from build123d import *

# Parameters (mm, degrees)
RESSALTO_EXTRUS_O1_DEPTH = 2
ESBO_O4_R                = 2.5
RESSALTO_EXTRUS_O2_DEPTH = 2
ESBO_O2_R                = 0.85
CORTE_EXTRUS_O1_DEPTH    = 17.680827318
CORTE_EXTRUS_O2_REACH    = 18.317
ESBO_O3_R                = 0.5
RESSALTO_EXTRUS_O3_DEPTH = 0.5


with BuildPart() as part:
    # Esboço1 → Ressalto-extrusão1 (new body)
    with BuildSketch(Plane(origin=(0, 0, 0), x_dir=(1, 0, 0), z_dir=(0, 1, 0))):
        with BuildLine():
            Line((-13.5, 2.5), (13.5, 2.5))
            ThreePointArc((13.5, 2.5), (16, 0), (13.5, -2.5))
            Line((13.5, -2.5), (-13.5, -2.5))
            ThreePointArc((-13.5, -2.5), (-16, 0), (-13.5, 2.5))
        make_face()
    extrude(amount=RESSALTO_EXTRUS_O1_DEPTH)

    # Esboço4 → Ressalto-extrusão2 (add)
    with BuildSketch(Plane(origin=(0, 2, 0), x_dir=(1, 0, 0), z_dir=(0, 1, 0))):
        with Locations(Location((-13.5, 0, 0), (0, 0, 270))):
            Circle(ESBO_O4_R)
    extrude(amount=RESSALTO_EXTRUS_O2_DEPTH)

    # Esboço2 → Corte-extrusão1 (cut, through all)
    with BuildSketch(Plane(origin=(0, 4, 0), x_dir=(1, 0, 0), z_dir=(0, 1, 0))):
        with Locations(Location((-13.5, 0, 0), (0, 0, 270))):
            Circle(ESBO_O2_R)
    extrude(amount=-CORTE_EXTRUS_O1_DEPTH, mode=Mode.SUBTRACT)

    # Esboço3 → Corte-extrusão2 (cut, up to next)
    with BuildSketch(Plane(origin=(0, 2, 0), x_dir=(1, 0, 0), z_dir=(0, 1, 0)), mode=Mode.PRIVATE) as corte_extrus_o2_sk1:
        with Locations(Location((13.5, 0, 0), (0, 0, 270))):
            Circle(ESBO_O3_R)
    corte_extrus_o2_tool1 = extrude(corte_extrus_o2_sk1.sketch, amount=-CORTE_EXTRUS_O2_REACH, mode=Mode.PRIVATE) & part.part
    add(corte_extrus_o2_tool1.solids().sort_by_distance((13.5, 2, 0))[0], mode=Mode.SUBTRACT)

    # Esboço5 → Ressalto-extrusão3 (add)
    with BuildSketch(Plane(origin=(0, 2, 0), x_dir=(1, 0, 0), z_dir=(0, 1, 0))):
        with BuildLine():
            Line((-10.245767212, -1), (-10.245767212, 1))
            Line((-10.245767212, 1), (-9.841921058, 1))
            add(Edge.make_bspline(
                [(-9.841921058, 1), (-9.806795922, 0.999747103), (-9.738934342, 0.999258507), (-9.640870086, 0.996160569), (-9.550136507, 0.990680303), (-9.467032017, 0.982697717), (-9.391328467, 0.972895983), (-9.323237834, 0.960610038), (-9.262408038, 0.946102512), (-9.224996929, 0.933733683), (-9.207305673, 0.927884615)],
                knots=[0, 0, 0, 0, 1.314313732, 2.53924729, 3.670748893, 4.714932338, 5.66265055, 6.526160246, 7.303039223, 8, 8, 8, 8], degree=3))
            add(Edge.make_bspline(
                [(-9.207305673, 0.927884615), (-9.184165822, 0.919067069), (-9.138410855, 0.90163193), (-9.073263928, 0.868742615), (-9.011935149, 0.831477985), (-8.954095638, 0.789788921), (-8.901066594, 0.742495007), (-8.850776368, 0.691605244), (-8.80528224, 0.63526905), (-8.763620356, 0.574654771), (-8.726057122, 0.510476455), (-8.693406175, 0.442856393), (-8.666289607, 0.372137989), (-8.643779192, 0.298517904), (-8.626038359, 0.22183426), (-8.613934398, 0.141997765), (-8.605950975, 0.059323942), (-8.60514866, 0.003224249), (-8.604741571, -0.025240385)],
                knots=[0, 0, 0, 0, 0.984719456, 1.947108742, 2.898477687, 3.838006223, 4.779231079, 5.722358779, 6.681677486, 7.655904652, 8.64651281, 9.637519902, 10.640069247, 11.656948941, 12.698408672, 13.768548281, 14.867775369, 16, 16, 16, 16], degree=3))
            add(Edge.make_bspline(
                [(-8.604741571, -0.025240385), (-8.605100981, -0.049961092), (-8.605809236, -0.098675829), (-8.612168845, -0.170470626), (-8.621412456, -0.240135524), (-8.635723426, -0.307338781), (-8.653096291, -0.372669192), (-8.675361521, -0.435430474), (-8.700867518, -0.496198365), (-8.730610306, -0.554151209), (-8.763262526, -0.609055993), (-8.798303522, -0.660813437), (-8.83569592, -0.708684993), (-8.875796281, -0.752815628), (-8.918086405, -0.793138816), (-8.962843165, -0.829991396), (-9.010182051, -0.862652284), (-9.059891036, -0.892404918), (-9.113420253, -0.918359407), (-9.171783605, -0.940319412), (-9.235229992, -0.958517478), (-9.303603682, -0.973700847), (-9.377022812, -0.98574502), (-9.455559364, -0.993817244), (-9.539092672, -0.999276063), (-9.596452252, -0.999754002), (-9.625975545, -1)],
                knots=[0, 0, 0, 0, 1.105936401, 2.179363191, 3.223086493, 4.248585256, 5.251745608, 6.245858792, 7.225916811, 8.198733463, 9.158002045, 10.082870192, 10.993790845, 11.873723703, 12.748670949, 13.606408763, 14.465103618, 15.319838547, 16.196477973, 17.123216899, 18.106603292, 19.147568657, 20.255746949, 21.433717677, 22.679120308, 24, 24, 24, 24], degree=3))
            Line((-9.625975545, -1), (-10.245767212, -1))
        make_face()
        with BuildLine():
            Line((-10.066280032, -0.794871795), (-9.836712725, -0.794871795))
            add(Edge.make_bspline(
                [(-9.836712725, -0.794871795), (-9.803725084, -0.794730026), (-9.740277771, -0.794457351), (-9.64904463, -0.792064664), (-9.565684974, -0.788154985), (-9.490186969, -0.782683512), (-9.422593241, -0.775444303), (-9.362762527, -0.76737293), (-9.31089095, -0.757317244), (-9.279502701, -0.74820241), (-9.264997981, -0.743990385)],
                knots=[0, 0, 0, 0, 1.375205317, 2.645023457, 3.804390687, 4.853969522, 5.800190428, 6.637939096, 7.370582563, 8, 8, 8, 8], degree=3))
            add(Edge.make_bspline(
                [(-9.264997981, -0.743990385), (-9.246741774, -0.737560923), (-9.21066541, -0.724855567), (-9.158733361, -0.70167976), (-9.110300787, -0.674227149), (-9.064523629, -0.643711564), (-9.022051255, -0.609056706), (-8.982380331, -0.57101614), (-8.945590731, -0.529396269), (-8.912062555, -0.484248748), (-8.882057809, -0.435854579), (-8.85607425, -0.384689531), (-8.833301946, -0.331314211), (-8.815428464, -0.274908978), (-8.801419559, -0.215978087), (-8.79149688, -0.154517394), (-8.785317038, -0.090538376), (-8.78459621, -0.047022876), (-8.78422875, -0.024839744)],
                knots=[0, 0, 0, 0, 0.998632004, 1.973411704, 2.929992603, 3.868527914, 4.809262121, 5.754881198, 6.702106254, 7.672490631, 8.653608572, 9.636854334, 10.631411391, 11.644891563, 12.686317036, 13.754757253, 14.855430412, 16, 16, 16, 16], degree=3))
            add(Edge.make_bspline(
                [(-8.78422875, -0.024839744), (-8.784522057, -0.001449183), (-8.785098262, 0.044501779), (-8.792340725, 0.111925034), (-8.802924471, 0.17677112), (-8.818229434, 0.239044374), (-8.837732794, 0.29886629), (-8.862072589, 0.35590601), (-8.889882086, 0.410765935), (-8.922969707, 0.462179858), (-8.959207189, 0.510804492), (-8.99942312, 0.555350158), (-9.04297857, 0.595918329), (-9.089398484, 0.633140794), (-9.139991112, 0.665520037), (-9.19356465, 0.694483855), (-9.250905033, 0.719064364), (-9.290798003, 0.732138), (-9.311071699, 0.738782051)],
                knots=[0, 0, 0, 0, 1.122418816, 2.205001699, 3.251619955, 4.274784885, 5.280384055, 6.268708349, 7.249350384, 8.229342522, 9.199999885, 10.157847722, 11.105861043, 12.055065948, 13.010012805, 13.98527497, 14.976112212, 16, 16, 16, 16], degree=3))
            add(Edge.make_bspline(
                [(-9.311071699, 0.738782051), (-9.327843783, 0.74342001), (-9.363505834, 0.753281583), (-9.421699814, 0.764038939), (-9.487194185, 0.773527224), (-9.560279728, 0.781560389), (-9.640873134, 0.787324573), (-9.729036384, 0.791651038), (-9.824807586, 0.794569114), (-9.891197606, 0.794768375), (-9.925655032, 0.794871795)],
                knots=[0, 0, 0, 0, 0.674548936, 1.434276114, 2.292660221, 3.240891867, 4.284742987, 5.42552168, 6.663806718, 8, 8, 8, 8], degree=3))
            Line((-9.925655032, 0.794871795), (-10.066280032, 0.794871795))
            Line((-10.066280032, 0.794871795), (-10.066280032, -0.794871795))
        make_face(mode=Mode.SUBTRACT)
    extrude(amount=RESSALTO_EXTRUS_O3_DEPTH)


solid = part.part
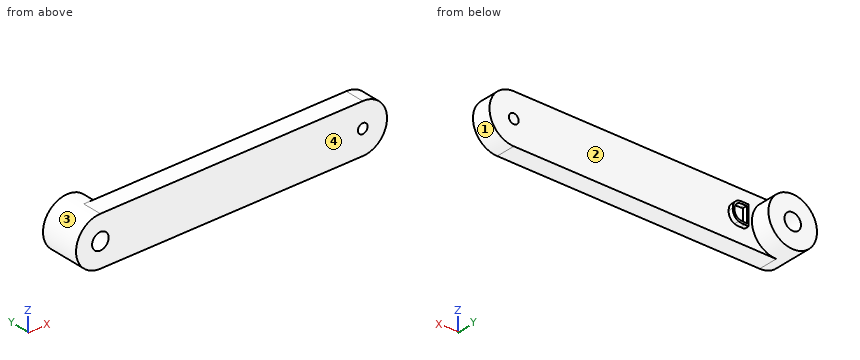
Input: part model. Units: mm. Frame: model coordinates. Face numbers are marked on the shaded views. A direction names the side the tool comes from. Give positions to 0.01 mm unless a question says otherwise; leave off trailing zeros. Loops run counter-clockwise (first coordinate to the right, second up) from the corner with the lowest first, then second, coordinate; pieces in that order, holes last. Notation, with made-up numbers: (-17, 56.5) -> (-4, 56.5) arc R30 cw to (-4, 89.5) -> close; hole circle Ø7 at (77, 46.25). An arc over 180 degrees is marked (long way). Answer as a JSON object with one key per item and string values. Group by question number.
Item 1: Cut plane A-A, the plane y = 1.3. Return the cut outline in (x, z), and give its area (3 significant figures).
Item 2: Reachability of the marked faces 3 and 4 from +Z, -Z, +X, -X, +Y, -Y: full face, straight path, thin tool, end or side. Return the list, or none.
Item 3: Pull-direction query (Z, two-part tool) for the marked faces 1 and 2; classes: released by +Z, released by -Z, zero draft, split by the parting line, or undercut.
Item 4: Line query: probe 1 along X at (y, z) = (2.25, 0); probe 2 along X at (y, z) = (1.7, 0); probe 3 along X at (y, z) = (3.25, 0). Output: solid intervals per line, ascending.
Item 5: Cut plane B-B, the plane z = 1.3. Return the cut outline in (x, y), and give its area (3 significant figures).
Item 6: Cut plane C-C, the plane y = 3.35. Return the cut outline in (x, z).
Item 7: Cut plane D-D, the plane x = -6. Return the cut outline in (y, z), and give its area (3 significant figures).
Item 8: Pin query (flat end, axial travel): P1, Ø1, axis at x = -9.5, z = 0, coming from the +Y side; P2, Ø1.8, axis at x = -9.5, z = 0.5, coming from the +Y side. Return the tip coordinate at first contact, or that it passes through.
Checks:
{
 "1": {"outline": "(-13.5, -2.5) -> (13.5, -2.5) arc R2.5 ccw to (13.5, 2.5) -> (-13.5, 2.5) arc R2.5 ccw to start; hole circle Ø1.7 at (-13.5, 0); hole circle Ø1 at (13.5, 0)", "area": "152 mm²"},
 "2": {"face 3": "+Y", "face 4": "+Z, -Z, +X, -X, -Y"},
 "3": {"face 1": "split by the parting line", "face 2": "zero draft"},
 "4": {"probe 1": "x = -16 to -14.35, -12.65 to -11, -10.25 to -10.07, -8.78 to -8.61", "probe 2": "x = -16 to -14.35, -12.65 to 13, 14 to 16", "probe 3": "x = -16 to -14.35, -12.65 to -11"},
 "5": {"outline": "(-15.64, 0) -> (15.64, 0) -> (15.64, 2) -> (-11.36, 2) -> (-11.36, 4) -> (-15.64, 4) -> close", "area": "71.1 mm²"},
 "6": {"outline": "circle Ø5 at (-13.5, 0); hole circle Ø1.7 at (-13.5, 0)"},
 "7": {"outline": "(0, -2.5) -> (2, -2.5) -> (2, 2.5) -> (0, 2.5) -> close", "area": "10.0 mm²"},
 "8": {"P1": "stops at y = 2", "P2": "stops at y = 2.5"}
}
